```python
from build123d import *

# Parameters (mm, degrees)
F3_DEPTH = 4
F4_SIZE  = 0.5


with BuildPart() as f1:
    # F0 (on Right) → F1 (revolve)
    with BuildSketch(Plane.YZ):
        with BuildLine():
            Line((0, 0), (0, 4))
            ThreePointArc((0, 4), (-2.828427, 2.828427), (-4, 0))
            Line((-4, 0), (0, 0))
        make_face()
    revolve(axis=Axis((0, 0, 2), (0, 0, -1)))

    # F2 (on face) → F3 (join)
    with BuildSketch(Plane(origin=(0, 0, 0), x_dir=(1, 0, 0), z_dir=(0, 0, -1))):
        Polygon((-0.142033, -5.773503), (4.928983, -3.009756), (5.071017, 2.763747), (0.142033, 5.773503), (-4.928983, 3.009756), (-5.071017, -2.763747), align=None)
    extrude(amount=F3_DEPTH)

    # F4
    f4_edges = [f1.edges().sort_by_distance(p)[0] for p in [
        (2.606525, -4.268625, 0),
        (5, 0.123005, 0),
        (2.393475, 4.391629, 0),
        (2.606525, -4.268625, -4),
        (-2.393475, -4.391629, -4),
        (-2.393475, -4.391629, 0),
        (-2.606525, 4.268625, 0),
        (-5, -0.123005, 0),
        (2.393475, 4.391629, -4),
        (-2.606525, 4.268625, -4),
        (5, 0.123005, -4),
        (-5, -0.123005, -4),
    ]]
    chamfer(f4_edges, length=F4_SIZE)


solid = f1.part
```
Verification items for the finished model (mm, model axes). A direction names the side the tool comes from. Round coordinates to 2 decimals unless told otherwise and drop trailing zeros. Order: outer loops, then holes, each group sorted by start corner. A loop starts at its lowest first (then second) coordinate and runs counter-clockwise, first axis right, second up. Notation, with made-up numbers: (87.25, -21) - (100.25, -21) arc R12 ccw to (100.25, -6) - close; hole circle Ø5 at (-38.75, 73). An arc over 180 degrees is marked (long way). Use CSV: the item, a comma, the result in double quotes. Start each with the question number.
1) Section check B-B, the plane y = 5. Record the cut outline in (x, z), plus the area to 3 significant figures.
2) Go/stop test with flat-tipped pins: P1, Ø3, axis at x = 1, y = -3.5, coming from the +Z side; P2, Ø1, axis at y = -3.5, z = 1.5, coming from the +X side; P3, Ø1, axis at x = -1, z = -1, coming from the +Y side. Record where each tip stops, or that it passes through.
3) Section check A-A, the plane z = -1.75. Record the cut outline in (x, y).
4) Access from +Z, -Z, +X, -X, +Y, -Y to the whole of each face (thin tool, end or side, straight path). Record for faces 1 (the flat face through (-4, 2, 0)), 2 (the flat face through (-2.509, 4.031, -3.754)).
5) Thickness scan on L1, parallel to Z at x = 3.75, y = 1.75; L2, parallel to X at y = 2.25, z = 2.75; L3, parallel to X at y = 1.5, z = 0.75. Record the ranges inside material, lowest first.
Answers:
1,outline,"(-1.41, -3.5) - (-0.45, -4) - (0.23, -4) - (1.28, -3.5) - (1.28, -0.5) - (0.23, 0) - (-0.45, 0) - (-1.41, -0.5) - close"
1,area,"9.74 mm²"
2,P1,"stops at z = 3.38"
2,P2,"stops at x = 2.25"
2,P3,"stops at y = 5.55"
3,outline,"(-5.07, 2.76) - (-4.93, -3.01) - (0.14, -5.77) - (5.07, -2.76) - (4.93, 3.01) - (-0.14, 5.77) - close"
4,face 1,"+Z"
4,face 2,"-Z, -X, +Y"
5,L1,"z = -4 to 0"
5,L2,"x = -1.84 to 1.84"
5,L3,"x = -3.63 to 3.63"
